from build123d import *

# Parameters (mm, degrees)
BOSS_EXTRUDE1_DEPTH = 10
SKETCH2_W           = 10
SKETCH2_H           = 10
BOSS_EXTRUDE2_DEPTH = 20
FILLET1_R           = 10


with BuildPart() as part:
    # Sketch1 → Boss-Extrude1 (new body)
    with BuildSketch(Plane(origin=(0, 0, 0), x_dir=(0, 0, -1), z_dir=(1, 0, 0))):
        Polygon((0, 0), (0, 80), (-10, 80), (-10, 10), (-50, 10), (-50, -50), (-10, -50), (-10, -100), (0, -100), (0, -40), (-40, -40), (-40, 0), align=None)
    extrude(amount=BOSS_EXTRUDE1_DEPTH)

    # Sketch2 → Boss-Extrude2 (add)
    with BuildSketch(Plane(origin=(10, 0, 0), x_dir=(0, 0, -1), z_dir=(1, 0, 0))):
        with Locations((-5, 75)):
            Rectangle(SKETCH2_W, SKETCH2_H)
        with Locations((-5, -95)):
            Rectangle(SKETCH2_W, SKETCH2_H)
    boss_extrude2 = extrude(amount=BOSS_EXTRUDE2_DEPTH)

    # Mirror1: Boss-Extrude2 across plane
    add(boss_extrude2.mirror(Plane.ZY.offset(-5)))

    # Fillet1
    fillet1_edges = [part.edges().sort_by_distance(p)[0] for p in [
        (10, -90, 5),
        (5, -40, 40),
        (0, -90, 5),
        (0, 70, 5),
        (5, -40, 0),
        (5, 0, 0),
        (10, 70, 5),
        (5, -50, 50),
        (5, 0, 40),
        (5, 10, 50),
        (5, -50, 10),
        (5, 10, 10),
    ]]
    fillet(fillet1_edges, radius=FILLET1_R)


solid = part.part
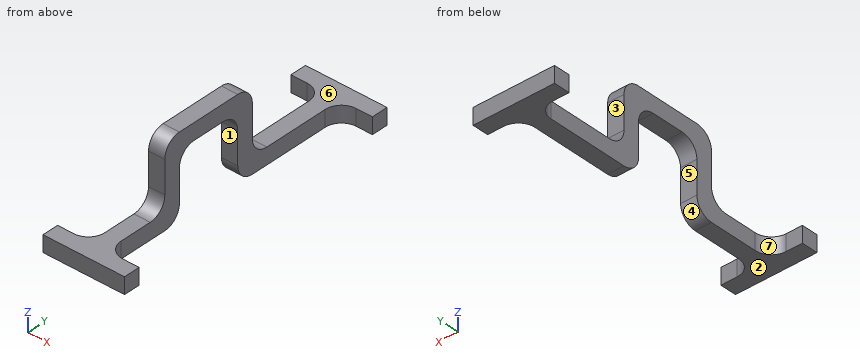
Work out the finished part from the listing and answer in its coordinate system (mm). Face numbers are marked on the shaded views. A direction names the side the tool comes from. Give positions to 0.01 mm unless a question says otherwise; leave off trailing zeros. Order: outer loops, then holes, each group sorted by start corner. A loop starts at its lowest first (then second) coordinate and runs counter-clockwise, first axis right, second up. Notation, with made-up numbers: (4, -12.75) -> (47, -12.75) arc R14 ccw to (47, -3.75) -> close; hole circle Ø2 at (79.25, 75.5). An arc over 180 degrees is marked (long way). Answer as a JSON object with one key per item and string values. Group by question number.
1. The mould has two halves that part along Y. Classify the marked faces 1, 2, 3 and 4: released by +Y, released by -Y, zero draft, split by the parting line, or undercut.
2. Section A-A on x = -16 is taken. Determine the outline of the cut face in (y, z), plus the area to 3 significant figures.
3. Section C-C on x = 4 is taken. Determine the outline of the cut face in (y, z).
4. Section B-B on z = 35 is taken. Determine the outline of the cut face in (x, y), plus the area to 3 significant figures.
5. Consider line 1 along Y through (x, z) = (-13, 3); line 2 along Y through (x, z) = (12.5, 9.5); line 3 along X through (y, z) = (-26, 47.5). Determine where each line is inside the solid, lowest interval first. Write a range as [from, to].
6. A tool of negligible diameter and unlimited length cuts with its end or side. For the marked faces 5, 6 and 7, from which of +Z, -Z, +X, -X, +Y, -Y can it reach the whole face along a straight path? Write none if from no direction.
7. Section D-D on y = -66 is taken. Determine the outline of the cut face in (x, z), plus the area to 3 significant figures.
8. Flat-ended cylindrical pins translate along their axes: pin 1 Ø25 at (x, y) = (5, 65) entering from +Z; pin 2 Ø11 at (x, z) = (6.5, 28.5) entering from +Y; pin 3 Ø8 at (y, z) = (43.5, 9.5) entering from -X. Find the tip coordinate at first contact, or state that the pin passes through.
Result sheet:
{
 "1": {"face 1": "undercut", "face 2": "zero draft", "face 3": "released by +Y", "face 4": "undercut"},
 "2": {"outline": "(-100, 0) -> (-90, 0) -> (-90, 10) -> (-100, 10) -> close; (70, 0) -> (80, 0) -> (80, 10) -> (70, 10) -> close", "area": "200 mm^2"},
 "3": {"outline": "(-100, 0) -> (-50, 0) arc R10 ccw to (-40, 10) -> (-40, 30) arc R10 cw to (-30, 40) -> (-10, 40) arc R10 cw to (0, 30) -> (0, 10) arc R10 ccw to (10, 0) -> (80, 0) -> (80, 10) -> (20, 10) arc R10 cw to (10, 20) -> (10, 40) arc R10 ccw to (0, 50) -> (-40, 50) arc R10 ccw to (-50, 40) -> (-50, 20) arc R10 cw to (-60, 10) -> (-100, 10) -> close"},
 "4": {"outline": "(0, -50) -> (10, -50) -> (10, -38.66) -> (0, -38.66) -> close; (0, -1.34) -> (10, -1.34) -> (10, 10) -> (0, 10) -> close", "area": "227 mm^2"},
 "5": {"line 1": "y = [-100, -90], [70, 80]", "line 2": "y = [-100, -86.61], [66.61, 80]", "line 3": "x = [0, 10]"},
 "6": {"face 5": "-Z, +X, -X", "face 6": "+Z, +X, -X, +Y", "face 7": "+Z, -Z, -X"},
 "7": {"outline": "(0, 0) -> (10, 0) -> (10, 10) -> (0, 10) -> close", "area": "100 mm^2"},
 "8": {"pin 1": "stops at z = 10", "pin 2": "stops at y = 10", "pin 3": "stops at x = 0"}
}
